Work out the finished part from the listing and answer in its coordinate system (mm). A direction names the side the tool comes from. Coordinates: 2 decimals unless noted, no trailing zeros. Order: outer loops, then holes, each group sorted by start corner. A loop starts at its lowest first (then second) coordinate and runs counter-clockwise, first axis right, second up. Notation, with made-up numbers: M -14.75,-29.75 L 29.25,-29.75 A25 ccw 29.25,-9.75 Z; hole C 57,-16.75 d3. An arc over 180 degrees is marked long. Use a Markdown table: item, result.
from build123d import *

# Parameters (mm, degrees)
EXTRUDE_1_DEPTH          = 3
CUT_EXTRUDE_2_DEPTH      = 29.442925307
CUT_EXTRUDE_2_DEPTH_BACK = 29.442925307
SKETCH_2_R               = 1.5
SKETCH_3_R               = 9.75
SKETCH_3_R_2             = 8.25
EXTRUDE_2_DEPTH          = 30
SKETCH_4_W               = 10.093928953
SKETCH_4_H               = 39.979180772
CUT_EXTRUDE_3_DEPTH      = 12.5
CUT_EXTRUDE_4_DEPTH      = 43.353932229
CUT_EXTRUDE_4_DEPTH_BACK = 43.353932229
SKETCH_5_R               = 1.5
SKETCH_6_R               = 2.25
CUT_EXTRUDE_5_DEPTH      = 1
CUT_EXTRUDE_6_DEPTH      = 1
FILLET_1_R               = 0.5


with BuildPart() as part:
    # Sketch 1 → Extrude 1 (new body)
    with BuildSketch(Plane.XY):
        with BuildLine():
            Line((-15, 20), (15, 20))
            ThreePointArc((15, 20), (18.535533906, 18.535533906), (20, 15))
            Line((20, 15), (20, -15))
            ThreePointArc((20, -15), (18.535533906, -18.535533906), (15, -20))
            Line((15, -20), (-15, -20))
            ThreePointArc((-15, -20), (-18.535533906, -18.535533906), (-20, -15))
            Line((-20, -15), (-20, 15))
            ThreePointArc((-20, 15), (-18.535533906, 18.535533906), (-15, 20))
        make_face()
    extrude(amount=EXTRUDE_1_DEPTH)

    # Sketch 2 → Cut-Extrude 2 (cut, two sides: drawn at the far end of the back side and taken through both)
    with BuildSketch(Plane.XY.offset(-CUT_EXTRUDE_2_DEPTH_BACK)):
        with Locations((-5.5, 14)):
            Circle(SKETCH_2_R)
        with Locations((5.5, 14)):
            Circle(SKETCH_2_R)
        with Locations((5.5, -14)):
            Circle(SKETCH_2_R)
        with Locations((-5.5, -14)):
            Circle(SKETCH_2_R)
    extrude(amount=CUT_EXTRUDE_2_DEPTH + CUT_EXTRUDE_2_DEPTH_BACK, mode=Mode.SUBTRACT)

    # Sketch 3 → Extrude 2 (add)
    with BuildSketch(Plane(origin=(0, 0, 0), x_dir=(1, 0, 0), z_dir=(0, -0.34202014332566943, 0.9396926207859081))):
        with Locations(Location((0, 0, 0), (0, 0, 64.109753518))):
            Circle(SKETCH_3_R)
        with Locations(Location((0, 0, 0), (0, 0, 90))):
            Circle(SKETCH_3_R_2, mode=Mode.SUBTRACT)
    extrude(amount=EXTRUDE_2_DEPTH)

    # Sketch 4 → Cut-Extrude 3 (cut, symmetric)
    with BuildSketch(Plane(origin=(0, 0, 0), x_dir=(0, 0, -1), z_dir=(1, 0, 0))):
        with Locations((5.046964477, 0.010409614)):
            Rectangle(SKETCH_4_W, SKETCH_4_H)
    extrude(amount=CUT_EXTRUDE_3_DEPTH, both=True, mode=Mode.SUBTRACT)

    # Sketch 5 → Cut-Extrude 4 (cut, two sides: drawn at the far end of the back side and taken through both)
    with BuildSketch(Plane(origin=(0, 0, 0), x_dir=(0, 0, -1), z_dir=(1, 0, 0)).offset(-CUT_EXTRUDE_4_DEPTH_BACK)):
        with Locations((-19.733545037, -7.18242301)):
            Circle(SKETCH_5_R)
    extrude(amount=CUT_EXTRUDE_4_DEPTH + CUT_EXTRUDE_4_DEPTH_BACK, mode=Mode.SUBTRACT)

    # Sketch 6 → Cut-Extrude 5 (cut)
    with BuildSketch(Plane(origin=(9.75, 0, 0), x_dir=(0, 0, -1), z_dir=(1, 0, 0))):
        with Locations((-19.733545037, -7.18242301)):
            Circle(SKETCH_6_R)
    extrude(amount=-CUT_EXTRUDE_5_DEPTH, mode=Mode.SUBTRACT)

    # Sketch 7 → Cut-Extrude 6 (cut)
    with BuildSketch(Plane(origin=(-9.75, 0, 0), x_dir=(0, 0, -1), z_dir=(1, 0, 0))):
        Polygon((-17.301027227, -9.223547807), (-16.749620205, -6.09636319), (-19.182138015, -4.055238393), (-22.166062846, -5.141298213), (-22.717469868, -8.26848283), (-20.284952058, -10.309607627), align=None)
    extrude(amount=CUT_EXTRUDE_6_DEPTH, mode=Mode.SUBTRACT)

    # Fillet 1
    fillet_1_edges = [part.edges().sort_by_distance(p)[0] for p in [
        (0, -18.013068421, 25.369112441),
    ]]
    fillet(fillet_1_edges, radius=FILLET_1_R)


solid = part.part
(1) Which of the six approach directions +Z, -Z, +X, -X, +Y, -Y give full straight-line access (tool end or side, diameter ignored) to faces 1 (the flat face through (0, 9, 3)), 2 (the cylindrical face through (-6.7, -14.9, 1.5)), 3 (the flat face through (-9.257, -9.275, 21.518))?
Conclusion:
| item | result |
|---|---|
| face 1 | none |
| face 2 | -Z |
| face 3 | -X |
(2) Straight lines are drawn through the part: L1, parallel to X at y = 14, z = 1.7; L2, parallel to Y at x = 5.5, z = 1.1; L3, parallel to Z at x = 13.5, y = -4.5. For each, find the intervals that lie inside material, in ascending order.
Conclusion:
| item | result |
|---|---|
| L1 | -20 to -7, -4 to 4, 7 to 20 |
| L2 | -20 to -15.5, -12.5 to 12.5, 15.5 to 20 |
| L3 | 0 to 3 |
(3) Given P1, Ø2.5, axis at x = 5.5, y = 14, coming from the -Z side; P2, Ø3.5, axis at x = -5.5, y = 14, coming from the +Z side; P3, Ø3, axis at y = -8, z = 20, coming from the -X side; P4, Ø3.5, axis at y = -7.18, z = 19.73, coming from the +X side, each flat-ended and moving along its own axis, determine where each tip first touches the part or whether it passes through.
Conclusion:
| item | result |
|---|---|
| P1 | through |
| P2 | z = 3 |
| P3 | x = -8.75 |
| P4 | x = 8.75 |
(4) A cutting plane is placed at A-A (y = 14). Determine the outline of the cut face in (x, z).
Conclusion:
| item | result |
|---|---|
| outline | M -20,0 L -7,0 L -7,3 L -20,3 Z; M -4,0 L 4,0 L 4,3 L -4,3 Z; M 7,0 L 20,0 L 20,3 L 7,3 Z |
(5) A cutting plane is placed at B-B (x = -5.5). Give the number of separate pieces and of enclosed holes in the cut face, then the cut area to 3 significant figures.
Conclusion:
| item | result |
|---|---|
| separate pieces | 3 |
| enclosed holes | 0 |
| area | 204 mm2 |
(6) A cutting plane is placed at C-C (x = 10.5). Determine the outline of the cut face in (y, z).
Conclusion:
| item | result |
|---|---|
| outline | M -20,0 L 20,0 L 20,3 L -20,3 Z |
(7) Determine the mould class of faces 4 (the flat face through (0, 0, 0)), 5 (the flat face through (-9.15, -7.68, 17.03)), 6 (the cylindrical face through (4.3, -14.9, 1.5)), 7 (the flat face through (8.75, -9, 19)) for opening direction Z: pulls with the +Z half, pulls with the -Z half, needs draft (parallel to the pull), parting line crosses it, or undercut.
Conclusion:
| item | result |
|---|---|
| face 4 | pulls with the -Z half |
| face 5 | undercut |
| face 6 | needs draft |
| face 7 | undercut |
